The listing builds one solid part. Answer for the finished solid, in the listing's coordinates (mm). Face numbers are marked on the shaded views. A direction names the side the tool comes from. Coordinates: 2 decimals unless noted, no trailing zeros. Loops run counter-clockwise (first coordinate to the right, second up) from the corner with the lowest first, then second, coordinate; pieces in that order, holes last. Notation, with made-up numbers: (23.25, 46) - (51.25, 46) arc R11 cw to (51.25, 64) - close; hole circle Ø11 at (41, 20). An arc over 180 degrees is marked (long way). Put each result on its own line as item: value.
```python
from build123d import *

# Parameters (mm, degrees)
BOSS_EXTRUDE1_DEPTH = 2.54
SKETCH2_W           = 31.75
SKETCH2_H           = 63.5
CUT_EXTRUDE1_DEPTH  = 48.268062421
SKETCH3_R           = 6.35
BOSS_EXTRUDE2_DEPTH = 12.7


with BuildPart() as part:
    # Sketch1 → Boss-Extrude1 (new body)
    with BuildSketch(Plane.XY):
        Polygon((-19.05, -34.925), (19.05, -34.925), (31.75, -34.925), (31.75, -22.225), (19.05, -22.225), (19.05, 34.925), (-19.05, 34.925), align=None)
    extrude(amount=BOSS_EXTRUDE1_DEPTH)

    # Sketch2 → Cut-Extrude1 (cut, through all)
    with BuildSketch(Plane.XY.offset(2.54)):
        Rectangle(SKETCH2_W, SKETCH2_H)
    extrude(amount=-CUT_EXTRUDE1_DEPTH, mode=Mode.SUBTRACT)

    # Sketch3 → Boss-Extrude2 (add)
    with BuildSketch(Plane.XY.offset(2.54)):
        with Locations((25.4, -28.575)):
            Circle(SKETCH3_R)
    extrude(amount=BOSS_EXTRUDE2_DEPTH)


solid = part.part
```
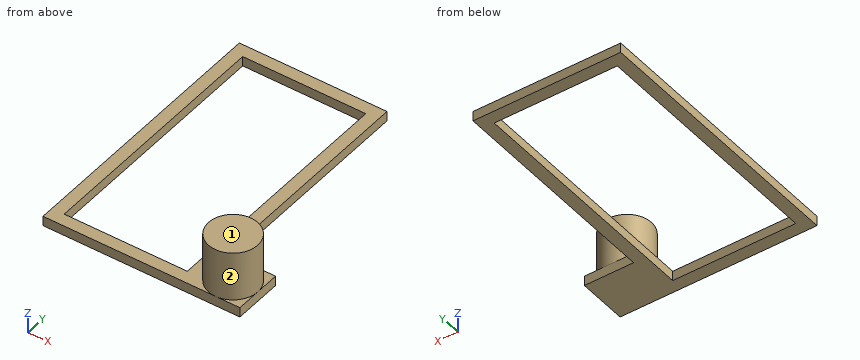
1) The part is cut by section C-C (x = 17). Give the vertices of the cut face in (y, z) (3 decimals), and give its area (3 significant figures).
Found:
outline: (-34.925, 0) - (34.925, 0) - (34.925, 2.54) - (-34.925, 2.54) - close
area: 177 mm^2
2) The part is cut by section B-B (y = 24.5). Give the vertices of the cut face in (x, z) (3 decimals).
Found:
outline: (-19.05, 0) - (-15.875, 0) - (-15.875, 2.54) - (-19.05, 2.54) - close; (15.875, 0) - (19.05, 0) - (19.05, 2.54) - (15.875, 2.54) - close
3) For the marked faces 1 and 2, determine the directions among +Z, -Z, +X, -X, +Y, -Y from which every point of the face is accessible in a straight line to the end or side of a thin tool.
Found:
face 1: +Z, +X, -X, +Y, -Y
face 2: +Z
4) The part is cut by section A-A (x = 5). Give the vertices of the cut face in (y, z) (3 decimals), and give its area (3 significant figures).
Found:
outline: (-34.925, 0) - (-31.75, 0) - (-31.75, 2.54) - (-34.925, 2.54) - close; (31.75, 0) - (34.925, 0) - (34.925, 2.54) - (31.75, 2.54) - close
area: 16.1 mm^2
5) Each of these flat-tipped pins is pushed along its axis until it touches: pin 1 (22 mm diameter, centred on x = -3, y = -16, fed in from +Z); pin 2 (0.8 mm diameter, centred on y = -7.5, z = 1, fed in from +X); pin 3 (3 mm diameter, centred on x = 25, z = 1.5, fed in from +Y) (3 decimals). Where does it stop, or does it pass through?
Found:
pin 1: passes through
pin 2: stops at x = 19.05
pin 3: stops at y = -22.225
6) The part is cut by section D-D (y = -27). Give the vertices of the cut face in (x, z) (3 decimals), and give its area (3 significant figures).
Found:
outline: (-19.05, 0) - (-15.875, 0) - (-15.875, 2.54) - (-19.05, 2.54) - close; (15.875, 0) - (31.75, 0) - (31.75, 2.54) - (31.552, 2.54) - (31.552, 15.24) - (19.248, 15.24) - (19.248, 2.54) - (15.875, 2.54) - close
area: 205 mm^2
7) Straight lines are drawn through the part: L1, parallel to Y at x = -11.5, z = 2.5 (3 decimals); L2, parallel to Z at x = -16, y = -25; L3, parallel to X at y = -23.5, z = 3.5. For each, find the intervals that lie inside material, in ascending order. Write a range as [from, to].
Found:
L1: y = [-34.925, -31.75], [31.75, 34.925]
L2: z = [0, 2.54]
L3: x = [21.58, 29.22]
